```python
from build123d import *

# Parameters (mm, degrees)
BOSS_EXTRUDE1_DEPTH = 10
SKETCH2_W           = 6
SKETCH2_H           = 4
BOSS_EXTRUDE2_DEPTH = 5
SKETCH3_R           = 2.15
CUT_EXTRUDE1_DEPTH  = 12
SKETCH6_R           = 2.15
CUT_EXTRUDE4_DEPTH  = 7.3
CUT_EXTRUDE5_START  = -10
SKETCH4_W           = 7.6
SKETCH4_H           = 3.5
CUT_EXTRUDE5_DEPTH  = 6.5
SKETCH7_W           = 7.6
SKETCH7_H           = 3.5
CUT_EXTRUDE6_DEPTH  = 6.5
CUT_EXTRUDE7_DEPTH  = 7.5


with BuildPart() as part:
    # Sketch1 → Boss-Extrude1 (new body)
    with BuildSketch(Plane.XY):
        Polygon((0, 70.768728377), (0, 0), (33, 0), align=None)
    extrude(amount=BOSS_EXTRUDE1_DEPTH)

    # Sketch2 → Boss-Extrude2 (add)
    with BuildSketch(Plane(origin=(0, 0, 0), x_dir=(-1, 0, 0), z_dir=(0, -1, 0))):
        with Locations((-16.5, -5)):
            Rectangle(SKETCH2_W, SKETCH2_H)
    extrude(amount=BOSS_EXTRUDE2_DEPTH)

    # Sketch3 → Cut-Extrude1 (cut)
    with BuildSketch(Plane(origin=(0, 0, 0), x_dir=(-1, 0, 0), z_dir=(0, -1, 0))):
        with Locations(Location((-23.33, -6, 0), (0, 0, 180))):
            Circle(SKETCH3_R)
        with Locations(Location((-8.55, -6, 0), (0, 0, 180))):
            Circle(SKETCH3_R)
    extrude(amount=-CUT_EXTRUDE1_DEPTH, mode=Mode.SUBTRACT)

    # Sketch6 → Cut-Extrude4 (cut)
    with BuildSketch(Plane(origin=(27.10599556, 12.639733311, 0), x_dir=(0, 0, -1), z_dir=(0.9063077870366479, 0.422618261740704, 0))):
        with Locations(Location((-5, 9.053597363, 0), (0, 0, 90))):
            Circle(SKETCH6_R)
        with Locations(Location((-5, 39.053597363, 0), (0, 0, 90))):
            Circle(SKETCH6_R)
    extrude(amount=-CUT_EXTRUDE4_DEPTH, mode=Mode.SUBTRACT)

    # Sketch4 → Cut-Extrude5 (cut)
    with BuildSketch(Plane(origin=(0, 0, 0), x_dir=(-1, 0, 0), z_dir=(0, 0, -1)).offset(CUT_EXTRUDE5_START)):
        with Locations((-23.33, 5.001728642)):
            Rectangle(SKETCH4_W, SKETCH4_H)
    extrude(amount=CUT_EXTRUDE5_DEPTH, mode=Mode.SUBTRACT)

    # Sketch7 → Cut-Extrude6 (cut)
    with BuildSketch(Plane.XY.offset(10)):
        with Locations((8.567911565, 5.001728642)):
            Rectangle(SKETCH7_W, SKETCH7_H)
    extrude(amount=-CUT_EXTRUDE6_DEPTH, mode=Mode.SUBTRACT)

    # Sketch9 → Cut-Extrude7 (cut)
    with BuildSketch(Plane.XY.offset(10)):
        Polygon((7.880441317, 46.768813524), (6.246018546, 50.199361906), (3.357135698, 48.823005888), (6.625981241, 41.961909123), (9.514864089, 43.338265141), align=None)
        Polygon((18.980916312, 23.03825064), (20.55828213, 19.581096164), (22.135647949, 16.123941687), (19.224359969, 14.795633629), (16.069628331, 21.709942582), align=None)
    extrude(amount=-CUT_EXTRUDE7_DEPTH, mode=Mode.SUBTRACT)


solid = part.part
```
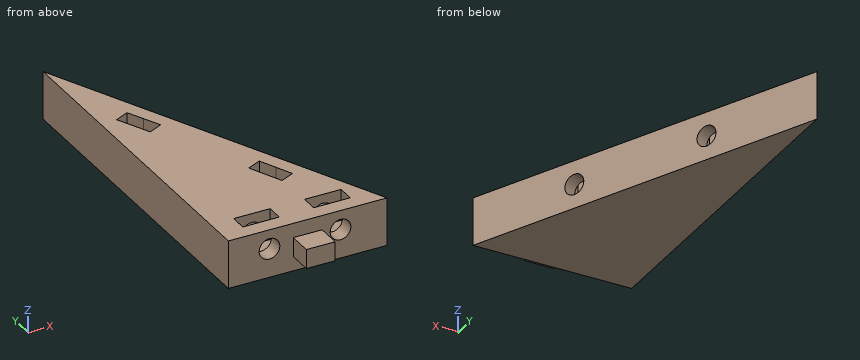
For this review, take the finished solid that the model builds, in its own axes (mm). Round coordinates to 2 decimals unless told otherwise and drop trailing zeros. Write each loop counter-clockwise with the first axis right and the second up, starting at its lowest first coordinate (ties: lowest second). Pieces come first, ordered by that corner, then holes. Notation, with made-up numbers: (45, -36) -> (70, -36) arc R27 ccw to (70, 1) -> close; hole circle Ø3 at (-4.75, 83.5). An arc over 180 degrees is marked (long way). One line per question, with ' | ' between items. Start each with the question number.
1) For pin 1 Ø6 at (x, z) = (8.5, 3.5) entering from -Y; pin 2 Ø2 at (x, y) = (11.5, 9) entering from -Z; pin 3 Ø2.5 at (x, z) = (23.33, 6) entering from +Y; pin 4 Ø1 at (x, y) = (9, 4) entering from +Z, all flat-tipped, find the tip position at first contact; note any pin that passes through.
2) Add section A-A (y = 55). Write out the cut boundary in (x, z), and give its area (3 significant figures).
3) Wall thickness on line 1 along Y through (x, z) = (7.5, 9.25); line 2 along Y through (x, z) = (5.5, 5.5); line 3 along Z through (x, y) = (8.55, 10.2): over which ranges is each line inside the solid? List them lowest first.
4) Add section B-B (z = 1.75). Write out the cut boundary in (x, y), and give its area (3 significant figures).
5) Add section C-C (y = 24.5). Write out the cut boundary in (x, z).
Reported:
1) pin 1: stops at y = 0 | pin 2: stops at z = 0 | pin 3: stops at y = 23.42 | pin 4: stops at z = 3.5
2) outline: (0, 0) -> (7.35, 0) -> (7.35, 10) -> (0, 10) -> close | area: 73.5 mm²
3) line 1: y = 0 to 3.25, 6.75 to 42.38, 47.57 to 54.68 | line 2: y = 0 to 3.25, 6.75 to 43.35, 49.84 to 58.97 | line 3: z = 0 to 3.85, 8.15 to 10
4) outline: (0, 0) -> (33, 0) -> (0, 70.77) -> close | area: 1,170 mm²
5) outline: (0, 0) -> (21.58, 0) -> (21.58, 10) -> (0, 10) -> close
